from build123d import *

# Parameters (mm, degrees)
SKETCH1_R                           = 2.38125
BOSS_EXTRUDE1_DEPTH                 = 7.62
MAGNET_START                        = 7.62
SKETCH1_3_R                         = 6.35
MAGNET_HOLE_DEPTH                   = 4.7752
CUT_EXTRUDE2_START                  = 7.62
CUT_EXTRUDE2_DEPTH                  = 5.6
F_3_0MM_DOWEL_HOLE1_D               = 3
F_3_0MM_DOWEL_HOLE1_DEPTH           = 9.106309071
F_3_0MM_DOWEL_HOLE1_TIP             = 0.901290929
F_3_0MM_DOWEL_HOLE1_ON_FACE_2_D     = 3
F_3_0MM_DOWEL_HOLE1_ON_FACE_2_DEPTH = 9.106309071
F_3_0MM_DOWEL_HOLE1_ON_FACE_2_TIP   = 0.901290929
F_3_0MM_DOWEL_HOLE1_ON_FACE_3_D     = 3
F_3_0MM_DOWEL_HOLE1_ON_FACE_3_DEPTH = 9.106309071
F_3_0MM_DOWEL_HOLE1_ON_FACE_3_TIP   = 0.901290929
F_3_0MM_DOWEL_HOLE1_ON_FACE_4_D     = 3
F_3_0MM_DOWEL_HOLE1_ON_FACE_4_DEPTH = 9.106309071
F_3_0MM_DOWEL_HOLE1_ON_FACE_4_TIP   = 0.901290929
F_3_0MM_DOWEL_HOLE1_ON_FACE_5_D     = 3
F_3_0MM_DOWEL_HOLE1_ON_FACE_5_DEPTH = 9.106309071
F_3_0MM_DOWEL_HOLE1_ON_FACE_5_TIP   = 0.901290929
F_3_0MM_DOWEL_HOLE2_D               = 3
F_3_0MM_DOWEL_HOLE2_DEPTH           = 13.2
CUT_EXTRUDE3_START                  = 7.62
CUT_EXTRUDE3_DEPTH                  = 3.175


with BuildPart() as part:
    # Sketch1 → Boss-Extrude1 (new body)
    with BuildSketch(Plane.XY):
        Polygon((44.45, 44.45), (9.731339272, 44.45), (0, 40.419147293), (0, 8.980256121), (-4.490128061, 4.490128061), (4.490128061, -4.490128061), (8.980256121, 0), (40.419147293, 0), (44.45, 9.731339272), align=None)
        with Locations(Location((15.869346859, 15.869346859, 0), (0, 0, 180))):
            Circle(SKETCH1_R, mode=Mode.SUBTRACT)
    extrude(amount=BOSS_EXTRUDE1_DEPTH)

    # Sketch1<3> → Magnet Hole (cut)
    with BuildSketch(Plane.XY.offset(MAGNET_START)):
        with Locations((15.869346859, 15.869346859)):
            Circle(SKETCH1_3_R)
    extrude(amount=-MAGNET_HOLE_DEPTH, mode=Mode.SUBTRACT)

    # Sketch1<4> → Cut-Extrude2 (cut)
    with BuildSketch(Plane.XY.offset(CUT_EXTRUDE2_START)):
        Polygon((36.580836926, 12.161131678), (34.917853767, 12.849961856), (31.473702876, 4.535046063), (33.136686034, 3.846215885), align=None)
        Polygon((6.151828996, 12.515790027), (12.515790027, 6.151828996), (13.788582233, 7.424621202), (7.424621202, 13.788582233), align=None)
        Polygon((12.161131678, 36.580836926), (12.849961856, 34.917853767), (4.535046063, 31.473702876), (3.846215885, 33.136686034), align=None)
    extrude(amount=-CUT_EXTRUDE2_DEPTH, mode=Mode.SUBTRACT)

    # Ø3.0mm Dowel Hole1
    with Locations(Plane(origin=(-1.414213562, 1.414213562, 4.87), x_dir=(-0.707106781187, 0.707106781187, 0), z_dir=(-0.707106781187, -0.707106781187, 0))):
        with Locations((1e-09, 0), (-3.999999999, 0)):
            Hole(F_3_0MM_DOWEL_HOLE1_D / 2, depth=F_3_0MM_DOWEL_HOLE1_DEPTH)
            with Locations((0, 0, -(F_3_0MM_DOWEL_HOLE1_DEPTH + F_3_0MM_DOWEL_HOLE1_TIP / 2))):  # 118° drill point
                Cone(0, F_3_0MM_DOWEL_HOLE1_D / 2, F_3_0MM_DOWEL_HOLE1_TIP, mode=Mode.SUBTRACT)

    # Ø3.0mm Dowel Hole1 on face 2
    with Locations(Plane(origin=(43.199940511, 6.713428701, 4.87), x_dir=(0.382682898036, 0.923879753837, 0), z_dir=(0.923879753837, -0.382682898036, 0))):
        with Locations((0, 0)):
            Hole(F_3_0MM_DOWEL_HOLE1_ON_FACE_2_D / 2, depth=F_3_0MM_DOWEL_HOLE1_ON_FACE_2_DEPTH)
            with Locations((0, 0, -(F_3_0MM_DOWEL_HOLE1_ON_FACE_2_DEPTH + F_3_0MM_DOWEL_HOLE1_ON_FACE_2_TIP / 2))):  # 118° drill point
                Cone(0, F_3_0MM_DOWEL_HOLE1_ON_FACE_2_D / 2, F_3_0MM_DOWEL_HOLE1_ON_FACE_2_TIP, mode=Mode.SUBTRACT)

    # Ø3.0mm Dowel Hole1 on face 3
    with Locations(Plane(origin=(41.669206782, 3.017910571, 4.87), x_dir=(0.382682898036, 0.923879753837, 0), z_dir=(0.923879753837, -0.382682898036, 0))):
        with Locations((0, 0)):
            Hole(F_3_0MM_DOWEL_HOLE1_ON_FACE_3_D / 2, depth=F_3_0MM_DOWEL_HOLE1_ON_FACE_3_DEPTH)
            with Locations((0, 0, -(F_3_0MM_DOWEL_HOLE1_ON_FACE_3_DEPTH + F_3_0MM_DOWEL_HOLE1_ON_FACE_3_TIP / 2))):  # 118° drill point
                Cone(0, F_3_0MM_DOWEL_HOLE1_ON_FACE_3_D / 2, F_3_0MM_DOWEL_HOLE1_ON_FACE_3_TIP, mode=Mode.SUBTRACT)

    # Ø3.0mm Dowel Hole1 on face 4
    with Locations(Plane(origin=(3.017910571, 41.669206782, 4.87), x_dir=(0.923879753837, 0.382682898036, 0), z_dir=(-0.382682898036, 0.923879753837, 0))):
        with Locations((0, 0)):
            Hole(F_3_0MM_DOWEL_HOLE1_ON_FACE_4_D / 2, depth=F_3_0MM_DOWEL_HOLE1_ON_FACE_4_DEPTH)
            with Locations((0, 0, -(F_3_0MM_DOWEL_HOLE1_ON_FACE_4_DEPTH + F_3_0MM_DOWEL_HOLE1_ON_FACE_4_TIP / 2))):  # 118° drill point
                Cone(0, F_3_0MM_DOWEL_HOLE1_ON_FACE_4_D / 2, F_3_0MM_DOWEL_HOLE1_ON_FACE_4_TIP, mode=Mode.SUBTRACT)

    # Ø3.0mm Dowel Hole1 on face 5
    with Locations(Plane(origin=(6.713428701, 43.199940511, 4.87), x_dir=(0.923879753837, 0.382682898036, 0), z_dir=(-0.382682898036, 0.923879753837, 0))):
        with Locations((0, 0)):
            Hole(F_3_0MM_DOWEL_HOLE1_ON_FACE_5_D / 2, depth=F_3_0MM_DOWEL_HOLE1_ON_FACE_5_DEPTH)
            with Locations((0, 0, -(F_3_0MM_DOWEL_HOLE1_ON_FACE_5_DEPTH + F_3_0MM_DOWEL_HOLE1_ON_FACE_5_TIP / 2))):  # 118° drill point
                Cone(0, F_3_0MM_DOWEL_HOLE1_ON_FACE_5_D / 2, F_3_0MM_DOWEL_HOLE1_ON_FACE_5_TIP, mode=Mode.SUBTRACT)

    # Ø3.0mm Dowel Hole2
    with Locations(Plane(origin=(0, 0, 0), x_dir=(-0.7071067811865495, 0.7071067811865457, 0), z_dir=(-0.7071067811865457, -0.7071067811865495, 0))):
        with Locations((-2, -4.87), (2, -4.87)):
            Hole(F_3_0MM_DOWEL_HOLE2_D / 2, depth=F_3_0MM_DOWEL_HOLE2_DEPTH)

    # Sketch1<5> → Cut-Extrude3 (cut)
    with BuildSketch(Plane.XY.offset(CUT_EXTRUDE3_START)):
        Polygon((5.960910165, 10.910657634), (1.958685784, 6.908433252), (6.908433252, 1.958685784), (10.910657634, 5.960910165), align=None)
        Polygon((2.118099231, 39.921854627), (4.284087459, 34.692696473), (10.751244186, 37.3714805), (8.585255959, 42.600638654), align=None)
        Polygon((37.3714805, 10.751244186), (42.600638654, 8.585255959), (39.921854627, 2.118099231), (34.692696473, 4.284087459), align=None)
    extrude(amount=-CUT_EXTRUDE3_DEPTH, mode=Mode.SUBTRACT)


solid = part.part
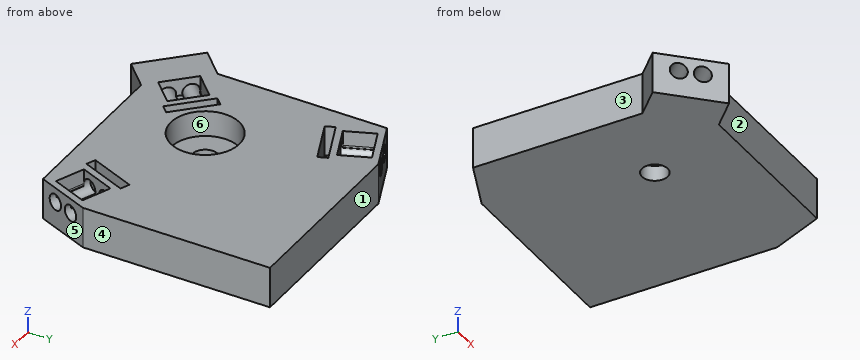
Could you check a few things on this model? Use its own coordinates, in mm. Face numbers are marked on the shaded views. A direction names the side the tool comes from. Give positions to 0.01 mm unless a question says otherwise; leave off trailing zeros. Write each loop counter-clockwise with the first axis right and the second up, starting at its lowest first coordinate (ties: lowest second). Pieces come first, ordered by that corner, then holes. Notation, with made-up numbers: (30.5, 88.25) -> (57.5, 88.25) arc R28 cw to (57.5, 121.25) -> close; hole circle Ø5 at (36, 20). An arc over 180 degrees is marked (long way). Answer as CSV lines item,"result". Start each with the question number.
(1) If we section it at C-C, the plane y = 3: Give the number of separate pieces and of enclosed holes in the cut face, and give its area (3 significant figures).
(2) If we section it at D-D, the plane x = 28: Write out the boundary of the cut face in (y, z).
(3) If we section it at A-A, the plane y = 17: Write out the boundary of the cut face in (x, z).
(4) If we mould it in two halves opening along Y, with no side actions, what happens to the marked faces 4, 5 and 6? For each: +Y half, -Y half, draft (parallel to the pull), parting line (faces both ways), or undercut.
(5) Please list where these lines run through material, in increasing order: line 1 (X direction, y = 8.5, z = 6.75); line 2 (X direction, y = 41, z = 4); line 3 (Y direction, x = 36.5, z = 5.75).
(6) I'm going to push flat-ended pins straight in: pin 1 Ø4 at (x, y) = (15.87, 15.87) entering from +Z; pin 2 Ø3.5 at (x, y) = (38.5, 7) entering from +Z (3 decimals); pin 3 Ø1.5 at (x, z) = (30.5, 6) entering from -Y. Where does each tip first touch, or does it pass through?
(7) Which directions (+Z, -Z, +X, -X, +Y, -Y) give clear straight access to the entire face, cutting with the end or side of a thin tool? Please do the marked faces 1, 2 and 3.
(8) If we section it at B-B, the plane x = 16: Write out the boundary of the cut face in (y, z), and give its area (3 significant figures).
Answer list:
1,separate pieces,"2"
1,enclosed holes,"1"
1,area,"304 mm^2"
2,outline,"(0, 0) -> (44.45, 0) -> (44.45, 7.62) -> (0, 7.62) -> close"
3,outline,"(0, 0) -> (13.77, 0) -> (13.77, 2.84) -> (9.62, 2.84) -> (9.62, 7.62) -> (0, 7.62) -> close; (17.97, 0) -> (44.45, 0) -> (44.45, 7.62) -> (22.12, 7.62) -> (22.12, 2.84) -> (17.97, 2.84) -> close"
4,face 4,"draft"
4,face 5,"-Y half"
4,face 6,"undercut"
5,line 1,"-0.48 to 3.55, 8.37 to 10.17, 12.71 to 33.12, 35.06 to 36.44, 42.57 to 43.94"
5,line 2,"1.4 to 1.97, 4.62 to 6.3, 8.95 to 44.45"
5,line 3,"0 to 3.54, 10.8 to 11.97, 12.19 to 44.45"
6,pin 1,"through"
6,pin 2,"z = 4.445"
6,pin 3,"y = 0"
7,face 1,"+Z, -Z, +X, -X, +Y"
7,face 2,"+Z, -Z, +X, -Y"
7,face 3,"+Z, -Z, -X, +Y"
8,outline,"(0, 0) -> (13.49, 0) -> (13.49, 2.84) -> (9.52, 2.84) -> (9.52, 7.62) -> (0, 7.62) -> close; (18.25, 0) -> (44.45, 0) -> (44.45, 7.62) -> (22.22, 7.62) -> (22.22, 2.84) -> (18.25, 2.84) -> close"
8,area,"265 mm^2"
